Model file for the job. Use its own axes, mm. Round coordinates to 2 decimals unless told otherwise and drop trailing zeros. Loops run counter-clockwise (first coordinate to the right, second up) from the corner with the lowest first, then second, coordinate; pieces in that order, holes last. Notation, with made-up numbers: M 30,-19.5 L 73,-19.5 A18 cw 73,15.5 Z; hole C 61.5,80.5 d11. An arc over 180 degrees is marked long. Use a Markdown table: item, result. Add a question column.
Item 1: Saw through at B-B on z = 55. Write the cut outline in (x, y) (3 decimals).
Item 2: Saw through at A-A on y = 6. Write the cut outline in (x, z) (3 decimals), then the cut area to 3 significant figures.
Item 3: Wall check: L1, parallel to Z at x = 0, y = -11.1; L2, parallel to Y at x = 5.25, z = 214 (3 decimals). Give the ranges that are in metal, low to high. Write a range as from..to.
```python
from build123d import *

# Parameters (mm, degrees)
SKETCH1_W           = 25.4
SKETCH1_H           = 25.4
SKETCH1_W_2         = 19.05
SKETCH1_H_2         = 19.05
BOSS_EXTRUDE1_DEPTH = 247.65
SKETCH2_R           = 1.5
CUT_EXTRUDE1_DEPTH  = 254
SKETCH3_R           = 1.5
CUT_EXTRUDE2_DEPTH  = 254


with BuildPart() as part:
    # Sketch1 → Boss-Extrude1 (new body)
    with BuildSketch(Plane.XY):
        Rectangle(SKETCH1_W, SKETCH1_H)
        Rectangle(SKETCH1_W_2, SKETCH1_H_2, mode=Mode.SUBTRACT)
    extrude(amount=BOSS_EXTRUDE1_DEPTH)

    # Sketch2 → Cut-Extrude1 (cut)
    with BuildSketch(Plane(origin=(12.7, 0, 0), x_dir=(0, 0, -1), z_dir=(1, 0, 0))):
        with Locations((-241.3, 0)):
            Circle(SKETCH2_R)
        with Locations((-6.35, 0)):
            Circle(SKETCH2_R)
    extrude(amount=-CUT_EXTRUDE1_DEPTH, mode=Mode.SUBTRACT)

    # Sketch3 → Cut-Extrude2 (cut)
    with BuildSketch(Plane(origin=(0, 12.7, 0), x_dir=(1, 0, 0), z_dir=(0, 1, 0))):
        with Locations((0, -12.7)):
            Circle(SKETCH3_R)
        with Locations((0, -234.95)):
            Circle(SKETCH3_R)
    extrude(amount=-CUT_EXTRUDE2_DEPTH, mode=Mode.SUBTRACT)


solid = part.part
```
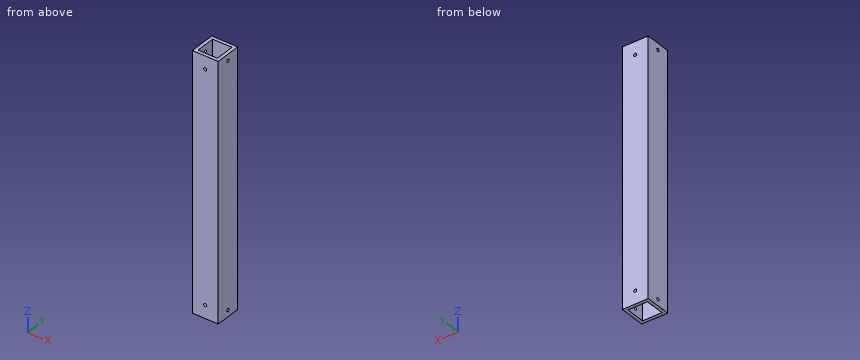
Entries:
| question | item | result |
|---|---|---|
| 1 | outline | M -12.7,-12.7 L 12.7,-12.7 L 12.7,12.7 L -12.7,12.7 Z; hole M -9.525,-9.525 L 9.525,-9.525 L 9.525,9.525 L -9.525,9.525 Z |
| 2 | outline | M -12.7,0 L -9.525,0 L -9.525,247.65 L -12.7,247.65 Z; M 9.525,0 L 12.7,0 L 12.7,247.65 L 9.525,247.65 Z |
| 2 | area | 1,570 mm2 |
| 3 | L1 | 0..11.2, 14.2..233.45, 236.45..247.65 |
| 3 | L2 | -12.7..-9.525, 9.525..12.7 |
